Can you work these out from the model? Positions are in its coordinate system, mm. A direction names the side the tool comes from. Give positions to 0.01 mm unless a question says otherwise; leave off trailing zeros. Order: outer loops, then holes, each group sorted by start corner. A loop starts at its lowest first (then second) coordinate and runs counter-clockwise, first axis right, second up.
```python
from build123d import *

# Parameters (mm, degrees)
SKETCH_1_W                           = 168
SKETCH_1_H                           = 168
SKETCH_1_W_2                         = 156
SKETCH_1_H_2                         = 156
EXTRUDE_1_DEPTH                      = 38
EXTRUDE_2_DEPTH                      = 15
SKETCH_3_R                           = 1.6
CUT_EXTRUDE_1_DEPTH                  = 122
PATTERN_CIRCULAR_1_COUNT             = 4
SKETCH_8_W                           = 20
SKETCH_8_H                           = 20
SKETCH_8_R                           = 2.6
EXTRUDE_3_DEPTH                      = 6
SKETCH_9_W                           = 20
SKETCH_9_H                           = 20
SKETCH_9_R                           = 2.6
EXTRUDE_4_DEPTH                      = 6
PATTERN_CIRCULAR_2_COUNT             = 4
SKETCH_10_W                          = 44
SKETCH_10_H                          = 7
EXTRUDE_5_DEPTH                      = 6
SKETCH_11_R                          = 1.55
CUT_EXTRUDE_3_DEPTH                  = 6
PATTERN_CIRCULAR_3_COUNT             = 2
PATTERN_CIRCULAR_3_ANGLE             = 90
SKETCH_12_R                          = 4.05
SKETCH_12_W                          = 44.3
SKETCH_12_H                          = 7.2
CUT_EXTRUDE_4_DEPTH                  = 6
SKETCH_16_R                          = 1.6
CUT_EXTRUDE_6_DEPTH                  = 6
PATTERN_CIRCULAR_4_COUNT             = 2
PATTERN_CIRCULAR_4_ANGLE             = 90
SKETCH_13_W                          = 12
SKETCH_13_H                          = 12
EXTRUDE_6_DEPTH                      = 6
SKETCH_15_R                          = 1.6
CUT_EXTRUDE_5_DEPTH                  = 6
CHAMFER_1_SIZE                       = 3
PATTERN_CIRCULAR_5_COUNT             = 4
CHAMFER_1_OF_PATTERN_CIRCULAR_5_SIZE = 3


with BuildPart() as part:
    # 草图1 → 凸台-拉伸1 (new body)
    with BuildSketch(Plane(origin=(0, 0, 0), x_dir=(1, 0, 0), z_dir=(0, 1, 0))):
        Rectangle(SKETCH_1_W, SKETCH_1_H)
        Rectangle(SKETCH_1_W_2, SKETCH_1_H_2, mode=Mode.SUBTRACT)
    extrude(amount=EXTRUDE_1_DEPTH)

    # 草图2 → 凸台-拉伸2 (add)
    with BuildSketch(Plane(origin=(0, 30, 0), x_dir=(1, 0, 0), z_dir=(0, 1, 0))):
        Polygon((-67.384062043, 63), (-78, 63), (-78, 78), (-63, 78), (-63, 67.384062043), align=None)
        Polygon((67.384062043, 63), (63, 67.384062043), (63, 78), (78, 78), (78, 63), align=None)
        Polygon((63, -67.384062043), (67.384062043, -63), (78, -63), (78, -78), (63, -78), align=None)
        Polygon((-67.384062043, -63), (-63, -67.384062043), (-63, -78), (-78, -78), (-78, -63), align=None)
    extrude(amount=-EXTRUDE_2_DEPTH)

    # 草图3 → 切除-拉伸1 (cut, through all)
    with BuildSketch(Plane(origin=(0, 15, 0), x_dir=(-1, 0, 0), z_dir=(0, -1, 0))):
        with Locations(Location((70.5, 70.5, 0), (0, 0, 90))):
            Circle(SKETCH_3_R)
    cut_extrude_1 = extrude(amount=-CUT_EXTRUDE_1_DEPTH, mode=Mode.SUBTRACT)

    # 阵列(圆周)1: 切除-拉伸1 ×4 about axis
    pattern_circular_1_axis = Axis((0, 0, 0), (0, 1, 0))
    for i in range(1, PATTERN_CIRCULAR_1_COUNT):
        add(cut_extrude_1.rotate(pattern_circular_1_axis, i * 360 / PATTERN_CIRCULAR_1_COUNT), mode=Mode.SUBTRACT)

    # 草图8 → 凸台-拉伸3 (add)
    with BuildSketch(Plane(origin=(0, 38, 0), x_dir=(1, 0, 0), z_dir=(0, 1, 0))):
        with Locations((-94, 74)):
            Rectangle(SKETCH_8_W, SKETCH_8_H)
        with Locations(Location((-94, 74, 0), (0, 0, 270))):
            Circle(SKETCH_8_R, mode=Mode.SUBTRACT)
    extrude_3 = extrude(amount=-EXTRUDE_3_DEPTH)

    # 草图9 → 凸台-拉伸4 (add)
    with BuildSketch(Plane(origin=(0, 38, 0), x_dir=(1, 0, 0), z_dir=(0, 1, 0))):
        with Locations((-74, 94)):
            Rectangle(SKETCH_9_W, SKETCH_9_H)
        with Locations(Location((-74, 94, 0), (0, 0, 270))):
            Circle(SKETCH_9_R, mode=Mode.SUBTRACT)
    extrude_4 = extrude(amount=-EXTRUDE_4_DEPTH)

    # 阵列(圆周)2: 凸台-拉伸3, 凸台-拉伸4 ×4 about axis
    pattern_circular_2_axis = Axis((0, 0, 0), (0, 1, 0))
    add([extrude_3.rotate(pattern_circular_2_axis, i * 360 / PATTERN_CIRCULAR_2_COUNT) for i in range(1, PATTERN_CIRCULAR_2_COUNT)])
    add([extrude_4.rotate(pattern_circular_2_axis, i * 360 / PATTERN_CIRCULAR_2_COUNT) for i in range(1, PATTERN_CIRCULAR_2_COUNT)])

    # 草图10 → 凸台-拉伸5 (add)
    with BuildSketch(Plane(origin=(0, 0, -84), x_dir=(-1, 0, 0), z_dir=(0, 0, -1))):
        with Locations((0, -3.5)):
            Rectangle(SKETCH_10_W, SKETCH_10_H)
    extrude_5 = extrude(amount=-EXTRUDE_5_DEPTH)

    # 草图11 → 切除-拉伸3 (cut)
    with BuildSketch(Plane(origin=(0, 0, -84), x_dir=(-1, 0, 0), z_dir=(0, 0, -1))):
        with Locations((-15.5, 30.5)):
            Circle(SKETCH_11_R)
        with Locations(Location((15.5, 30.5, 0), (0, 0, 180))):
            Circle(SKETCH_11_R)
        with Locations((15.5, -0.5)):
            Circle(SKETCH_11_R)
        with Locations(Location((-15.5, -0.5, 0), (0, 0, 180))):
            Circle(SKETCH_11_R)
        with BuildLine():
            Line((-5, -7), (-5, 9.409830056))
            ThreePointArc((-5, 9.409830056), (0, 22.5), (5, 9.409830056))
            Line((5, 9.409830056), (5, -7))
            Line((5, -7), (-5, -7))
        make_face()
    cut_extrude_3 = extrude(amount=-CUT_EXTRUDE_3_DEPTH, mode=Mode.SUBTRACT)

    # 阵列(圆周)3: 凸台-拉伸5, 切除-拉伸3 ×2 about axis
    pattern_circular_3_axis = Axis((0, 0, 0), (0, -1, 0))
    add([extrude_5.rotate(pattern_circular_3_axis, i * PATTERN_CIRCULAR_3_ANGLE / (PATTERN_CIRCULAR_3_COUNT - 1)) for i in range(1, PATTERN_CIRCULAR_3_COUNT)])
    add([cut_extrude_3.rotate(pattern_circular_3_axis, i * PATTERN_CIRCULAR_3_ANGLE / (PATTERN_CIRCULAR_3_COUNT - 1)) for i in range(1, PATTERN_CIRCULAR_3_COUNT)], mode=Mode.SUBTRACT)

    # 草图12 → 切除-拉伸4 (cut)
    with BuildSketch(Plane.XY.offset(84)):
        with Locations((0, 15)):
            Circle(SKETCH_12_R)
        with Locations((0, 3.6)):
            Rectangle(SKETCH_12_W, SKETCH_12_H)
    cut_extrude_4 = extrude(amount=-CUT_EXTRUDE_4_DEPTH, mode=Mode.SUBTRACT)

    # 草图16 → 切除-拉伸6 (cut)
    with BuildSketch(Plane.XY.offset(84)):
        with Locations((-20, 15)):
            Circle(SKETCH_16_R)
        with Locations(Location((20, 15, 0), (0, 0, 180))):
            Circle(SKETCH_16_R)
    cut_extrude_6 = extrude(amount=-CUT_EXTRUDE_6_DEPTH, mode=Mode.SUBTRACT)

    # 阵列(圆周)4: 切除-拉伸4, 切除-拉伸6 ×2 about axis
    pattern_circular_4_axis = Axis((0, 0, 0), (0, -1, 0))
    add([cut_extrude_4.rotate(pattern_circular_4_axis, i * PATTERN_CIRCULAR_4_ANGLE / (PATTERN_CIRCULAR_4_COUNT - 1)) for i in range(1, PATTERN_CIRCULAR_4_COUNT)], mode=Mode.SUBTRACT)
    add([cut_extrude_6.rotate(pattern_circular_4_axis, i * PATTERN_CIRCULAR_4_ANGLE / (PATTERN_CIRCULAR_4_COUNT - 1)) for i in range(1, PATTERN_CIRCULAR_4_COUNT)], mode=Mode.SUBTRACT)

    # 草图13 → 凸台-拉伸6 (add)
    with BuildSketch(Plane.XZ):
        with Locations((-72, 52)):
            Rectangle(SKETCH_13_W, SKETCH_13_H)
        with Locations((-52, 72)):
            Rectangle(SKETCH_13_W, SKETCH_13_H)
    extrude_6 = extrude(amount=-EXTRUDE_6_DEPTH)

    # 草图15 → 切除-拉伸5 (cut)
    with BuildSketch(Plane.XZ):
        with Locations(Location((-72, 52, 0), (0, 0, 270))):
            Circle(SKETCH_15_R)
        with Locations(Location((-52, 72, 0), (0, 0, 90))):
            Circle(SKETCH_15_R)
    cut_extrude_5 = extrude(amount=-CUT_EXTRUDE_5_DEPTH, mode=Mode.SUBTRACT)

    # 倒角1
    chamfer_1_edges = [part.edges().sort_by_distance(p)[0] for p in [
        (-66, 3, 58),
        (-66, 3, 46),
        (-46, 3, 66),
        (-58, 3, 66),
    ]]
    chamfer(chamfer_1_edges, length=CHAMFER_1_SIZE)

    # 阵列(圆周)5: 凸台-拉伸6, 切除-拉伸5 ×4 about axis
    pattern_circular_5_axis = Axis((0, 0, 0), (0, 1, 0))
    add([extrude_6.rotate(pattern_circular_5_axis, i * 360 / PATTERN_CIRCULAR_5_COUNT) for i in range(1, PATTERN_CIRCULAR_5_COUNT)])
    add([cut_extrude_5.rotate(pattern_circular_5_axis, i * 360 / PATTERN_CIRCULAR_5_COUNT) for i in range(1, PATTERN_CIRCULAR_5_COUNT)], mode=Mode.SUBTRACT)

    # 倒角1 of 阵列(圆周)5
    chamfer_1_of_pattern_circular_5_edges = [part.edges().sort_by_distance(p)[0] for p in [
        (58, 3, 66),
        (46, 3, 66),
        (66, 3, 46),
        (66, 3, 58),
        (66, 3, -58),
        (66, 3, -46),
        (46, 3, -66),
        (58, 3, -66),
        (-58, 3, -66),
        (-46, 3, -66),
        (-66, 3, -46),
        (-66, 3, -58),
    ]]
    chamfer(chamfer_1_of_pattern_circular_5_edges, length=CHAMFER_1_OF_PATTERN_CIRCULAR_5_SIZE)


solid = part.part
```
1) I'm going to push flat-ended pins straight in: pin 1 Ø3 at (x, z) = (52, 72) entering from -Y; pin 2 Ø2 at (y, z) = (31, 39.5) entering from -X; pin 3 Ø11.5 at (x, y) = (-26, 22) entering from -Z; pin 4 Ø16 at (x, z) = (95.5, 69) entering from -Y. Where does each tip first touch, or does it pass through?
2) Suppose I cut it at D-D (x = -94). Please give me the cut outline in (y, z).
3) We'd pull the mould along X, two halves only. Please class faces 4 (the face through (-72, 32, -96)), 5 (the face through (84, 35, -94)), 6 (the face through (73.4, 6, 53.4)): +X half, -X half, draft (parallel to the pull), parting line (faces both ways), or undercut.
4) Suppose I cut it at B-B (z = -30.5). Please give me the cut outline in (x, y), and give its area (3 significant figures).
5) Suppose I cut it at A-A (x = 11.5). Please give me the cut outline in (y, z), and give its area (3 significant figures).
6) Which directions (+Z, -Z, +X, -X, +Y, -Y) give clear straight access to the entire face, cutting with the end or side of a thin tool? Please do faces 1 (the face through (64, 35, -94)), 2 (the face through (66, 3, 52)), 3 (the face through (94, 35, 84)).
7) Suppose I cut it at C-C (z = 94). Please give me the cut outline in (x, y).
8) If I drill on line 1 (Y direction, x = 15.5, z = -82.7); line 2 (X direction, y = 2.75, z = 72); line 3 (X direction, y = 4.3, z = -52), over which ranges is the centre line in solid material (lowest first)?
Results:
1. pin 1: passes through
1. pin 2: stops at x = -84
1. pin 3: stops at z = -84
1. pin 4: stops at y = 32
2. outline: (32, -84) - (38, -84) - (38, -76.6) - (32, -76.6) - close; (32, -71.4) - (38, -71.4) - (38, -64) - (32, -64) - close; (32, 64) - (38, 64) - (38, 71.4) - (32, 71.4) - close; (32, 76.6) - (38, 76.6) - (38, 84) - (32, 84) - close
3. face 4: draft
3. face 5: +X half
3. face 6: undercut
4. outline: (-84, 0) - (-78, 0) - (-78, 38) - (-84, 38) - close; (78, 0) - (84, 0) - (84, 38) - (78, 38) - close
4. area: 456 mm2
5. outline: (-7, -84) - (38, -84) - (38, -78) - (-7, -78) - close; (7.2, 78) - (38, 78) - (38, 84) - (7.2, 84) - close
5. area: 455 mm2
6. face 1: -Z, +Y, -Y
6. face 2: +Y, -Y
6. face 3: +Z, +X, +Y, -Y
7. outline: (-84, 32) - (-76.6, 32) - (-76.6, 38) - (-84, 38) - close; (-71.4, 32) - (-64, 32) - (-64, 38) - (-71.4, 38) - close; (64, 32) - (71.4, 32) - (71.4, 38) - (64, 38) - close; (76.6, 32) - (84, 32) - (84, 38) - (76.6, 38) - close
8. line 1: y = -7 to -2.05, 1.05 to 28.95, 32.05 to 38
8. line 2: x = -84 to -78, -58 to -53.6, -50.4 to -46, 46 to 50.4, 53.6 to 58, 78 to 84
8. line 3: x = -84 to -73.6, -70.4 to -66, 66 to 70.4, 73.6 to 84
